Geometry: see drawing. Coordinates: mm, zero at the bounding-box minimum. A direction names the side the tool comes from. Give positions to 0.01 mm unless a question says otherwise; leave off trailing zeros. Return JSON: item names as keys, results as strings. Group by question number.
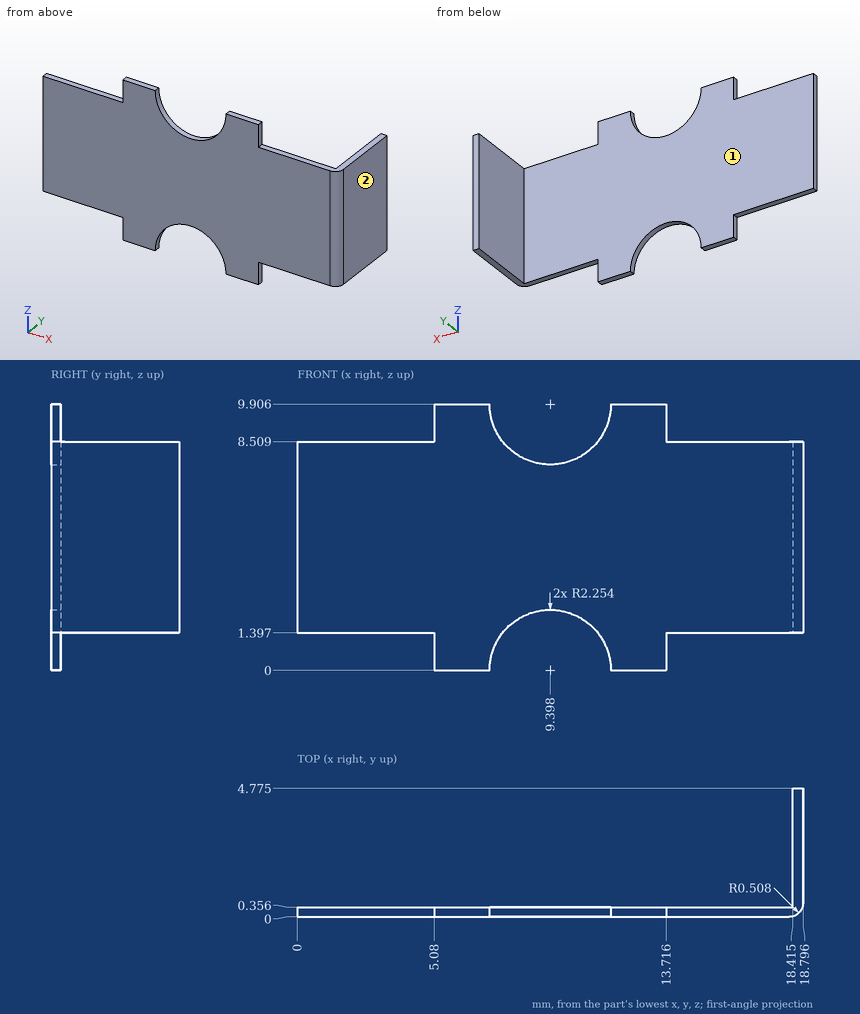
1) Material intervals for line 1 (X direction, y = 2.45, z = 5.25) (1 decimal); line 2 (Y direction, x = 7.25, z = 7) (1 decimal), sorted ascending.
2) Contact query for flat-ended pins moving along their axis: P1, Ø1.3, axis at y = 3, z = 4.5, coming from the -X side (3 decimals); P2, Ø3, axis at x = 9, z = 7, coming from the +Y side. Output: stop coordinate, or through.
3) Reachability of the marked faces 1 and 2 from +Z, -Z, +X, -X, +Y, -Y: full face, straight path, thin tool, end or side. Return the list, or none.
Calculated:
{
 "1": {"line 1": "18.4 to 18.8", "line 2": "0 to 0.4"},
 "2": {"P1": "x = 18.415", "P2": "y = 0.36"},
 "3": {"face 1": "+Z, -Z, -X, +Y", "face 2": "+Z, -Z, +X, +Y, -Y"}
}
